from build123d import *

# Parameters (mm, degrees)
F0_R     = 4.7625
F0_R_2   = 2.5527
F1_DEPTH = 6


with BuildPart() as f1:
    # F0 (on Top) → F1 (new body)
    with BuildSketch(Plane.XY):
        with BuildLine():
            Line((20.446472, 0), (-30.353528, 0))
            Line((-30.353528, 0), (-30.353528, -25.4))
            ThreePointArc((-30.353528, -25.4), (-4.953528, -50.8), (20.446472, -25.4))
            Line((20.446472, -25.4), (20.446472, 0))
        make_face()
        with Locations((-4.953528, -25.4)):
            Circle(F0_R, mode=Mode.SUBTRACT)
        with Locations((-24.003528, -8.3061)):
            Circle(F0_R_2, mode=Mode.SUBTRACT)
        with Locations((-11.303528, -8.3061)):
            Circle(F0_R_2, mode=Mode.SUBTRACT)
        with Locations((1.396472, -8.3061)):
            Circle(F0_R_2, mode=Mode.SUBTRACT)
        with Locations((14.096472, -8.3061)):
            Circle(F0_R_2, mode=Mode.SUBTRACT)
    extrude(amount=F1_DEPTH)


solid = f1.part
For this review, take the finished solid that the model builds, in its own axes (mm). Give positions to 0.01 mm unless a question says otherwise; leave off trailing zeros. Order: outer loops, then holes, each group sorted by start corner. A loop starts at its lowest first (then second) coordinate and runs counter-clockwise, first axis right, second up. Notation, with made-up numbers: (71, 61.25) - (75, 61.25) arc R21 ccw to (75, 77.25) - close; hole circle Ø11 at (75, 20). An arc over 180 degrees is marked (long way). Answer as a JSON object with one key per item and string values. Group by question number.
Item 1: Draft analysis for pull direction Y (two halves, no side actions). For faces 1 (the flat face through (-30.354, -13, 3)), 2 (the cylindrical face through (-5.512, -50.794, 2.958)), 3 (the cylindrical face through (-21.57, -7.54, 2.96)), 4 (the cylindrical face through (1.064, -5.775, 2.958)), state which applies: pulls with the +Y half, pulls with the -Y half, needs draft (parallel to the pull), parting line crosses it, or undercut.
Item 2: Take a section at C-C on z = 2.6. Give the boundary of the cut face in (x, y) (1 decimal), and give its area (3 significant figures).
Item 3: Take a section at D-D on x = 8.5. Give the boundary of the cut face in (y, z).
Item 4: Take a section at A-A on x = -24. Give the boundary of the cut face in (y, z), and give its area (3 significant figures).
Item 5: Wall thickness on line 1 along X through (y, z) = (-10, 5.15); line 2 along X through (y, z) = (-9, 4.3); line 3 along Y through (x, z) = (14, 4.6): over which ranges is each line inside the solid? List them lowest first.
Item 6: Take a section at B-B on y = -24.5. Give the boundary of the cut face in (x, z).
Item 7: Clearance check with flat-ended pins moving along their axes: pin 1 Ø6 at (x, y) = (6, -12.5) entering from -Z; pin 2 Ø8.5 at (x, y) = (-4.95, -25.4) entering from +Z. State where each tip first meets the part, or that it passes through.
Reported:
{
 "1": {"face 1": "needs draft", "face 2": "pulls with the -Y half", "face 3": "undercut", "face 4": "undercut"},
 "2": {"outline": "(-30.4, -25.4) arc R25.4 ccw to (20.4, -25.4) - (20.4, 0) - (-30.4, 0) - close; hole circle Ø5.1 at (-24, -8.3); hole circle Ø5.1 at (-11.3, -8.3); hole circle Ø9.5 at (-5, -25.4); hole circle Ø5.1 at (1.4, -8.3); hole circle Ø5.1 at (14.1, -8.3)", "area": "2,150 mm^2"},
 "3": {"outline": "(-46.94, 0) - (0, 0) - (0, 6) - (-46.94, 6) - close"},
 "4": {"outline": "(-42.2, 0) - (-10.86, 0) - (-10.86, 6) - (-42.2, 6) - close; (-5.75, 0) - (0, 0) - (0, 6) - (-5.75, 6) - close", "area": "223 mm^2"},
 "5": {"line 1": "-30.35 to -25.91, -22.09 to -13.21, -9.39 to -0.51, 3.31 to 12.19, 16.01 to 20.45", "line 2": "-30.35 to -26.46, -21.55 to -13.76, -8.85 to -1.06, 3.85 to 11.64, 16.55 to 20.45", "line 3": "-42.31 to -10.86, -5.76 to 0"},
 "6": {"outline": "(-30.35, 0) - (-9.63, 0) - (-9.63, 6) - (-30.35, 6) - close; (-0.28, 0) - (20.45, 0) - (20.45, 6) - (-0.28, 6) - close"},
 "7": {"pin 1": "z = 0", "pin 2": "through"}
}
